Autodesk Inventor part; units mm, degrees
ref_plane "YZ Plane" through (0, 0, 0) normal (1, 0, 0) x (0, 1, 0)
ref_plane "XZ Plane" through (0, 0, 0) normal (0, 1, 0) x (-1, 0, 0)
ref_plane "XY Plane" through (0, 0, 0) normal (0, 0, 1) x (1, 0, 0)
sketch "スケッチ1" plane through (0, 0, 0) normal (0, 0, 1) x (1, 0, 0)
  circle A0 centre (0, 0) radius 25
  dimension "d0" = 50
extrude "押し出し1" add sketch "スケッチ1" along normal blind 3
sketch "スケッチ2" plane through (0, 0, 3) normal (0, 0, 1) x (1, 0, 0)
  circle A0 centre (0, 0) radius 18.13
  dimension "d3" = 36.26
extrude "押し出し2" add sketch "スケッチ2" along normal blind 40
sketch "スケッチ3" plane through (0, 0, 43) normal (0, 0, 1) x (1, 0, 0)
  circle A0 centre (0, 0) radius 25
  dimension "d6" = 50
extrude "押し出し3" add sketch "スケッチ3" along normal blind 3
sketch "スケッチ4" plane through (0, 0, 46) normal (0, 0, 1) x (1, 0, 0)
  circle A0 centre (0, 0) radius 2.5
  dimension "d9" = 5
hole "穴1" at (0, 0, 46) direction (0, 0, -1) diameter 5 depth 46
equation "\"BendRadius\" = Thickness"
equation "\"BendReliefWidth\" = Thickness"
equation "\"BendReliefDepth\" = 0.5 * Thickness"
equation "\"CornerReliefSize\" = 4 * Thickness"
equation "\"MinimumRemnant\" = 2 * Thickness"
equation "\"TransitionRadius\" = BendRadius"
equation "\"JacobiRadiusSize\" = BendRadius"
equation "\"GapSize\" = Thickness"
properties part number "nhk12"
For this review, take the finished solid that the model builds, in its own axes (mm). A direction names the side the tool comes from. Round coordinates to 2 decimals unless told otherwise and drop trailing zeros. Order: outer loops, then holes, each group sorted by start corner. A loop starts at its lowest first (then second) coordinate and runs counter-clockwise, first axis right, second up.
Q1. Mouldability with a two-part tool opening along Z and no side actions: class faces 1 (the flat face through (0, -5, 0)), 2 (the cylindrical face through (23.846, -7.509, 44.479)), 3 (the flat face through (17, 8, 3)) as pulls with the +Z half, pulls with the -Z half, needs draft (parallel to the pull), parting line crosses it, or undercut.
Findings below:
face 1: pulls with the -Z half
face 2: needs draft
face 3: undercut
Q2. Wall thickness on line 1 (Z direction, x = -14.5, y = 16.5); line 2 (Y direction, x = 0, z = 32); line 3 (Y direction, x = 7, z = 12): over which ranges is each line inside the solid? List them lowest first.
Findings below:
line 1: z = 0 to 3, 43 to 46
line 2: y = -18.13 to -2.5, 2.5 to 18.13
line 3: y = -16.72 to 16.72
Q3. Insertion check: P1, Ø6, axis at x = 5.5, z = 34.5, coming from the +Y side; P2, Ø1, axis at x = 14, z = 5.5, coming from the -Y side; P3, Ø6, axis at x = 4.5, z = 35, coming from the +Y side. Each pin has a flat end and moves straight along its axis. Give the tip position at first contact, or say it passes through.
Findings below:
P1: stops at y = 17.96
P2: stops at y = -12.1
P3: stops at y = 18.07
Q4. Machinability: for faces 4 (the flat face through (17, 8, 43)), 5 (the cylindrical face through (2.44, 0.54, 22.68)), which of the approach directions +Z, -Z, +X, -X, +Y, -Y give a long, thin tool a straight path to every point of the face, cutting with its end or side? Answer none if there is none.
Findings below:
face 4: none
face 5: +Z, -Z
Q5. We need section A-A, the plane y = 0. Give the boundary of the cut face in (x, z), plus the area to 3 significant figures.
Findings below:
outline: (-25, 0) - (-2.5, 0) - (-2.5, 46) - (-25, 46) - (-25, 43) - (-18.13, 43) - (-18.13, 3) - (-25, 3) - close; (2.5, 0) - (25, 0) - (25, 3) - (18.13, 3) - (18.13, 43) - (25, 43) - (25, 46) - (2.5, 46) - close
area: 1,520 mm2
Q6. We need section D-D, the plane x = -6. Give the boundary of the cut face in (y, z).
Findings below:
outline: (-24.27, 0) - (24.27, 0) - (24.27, 3) - (17.11, 3) - (17.11, 43) - (24.27, 43) - (24.27, 46) - (-24.27, 46) - (-24.27, 43) - (-17.11, 43) - (-17.11, 3) - (-24.27, 3) - close
Q7. We need section C-C, the plane z = 24.5. Give the boundary of the cut face in (x, y).
Findings below:
outline: circle Ø36.26 at (0, 0); hole circle Ø5 at (0, 0)
